Verification items for the finished model (mm, model axes). A direction names the side the tool comes from. Coordinates: 2 decimals unless noted, no trailing zeros. Write each loop counter-clockwise with the first axis right and the second up, starting at its lowest first coordinate (ties: lowest second). Pieces come first, ordered by that corner, then holes. Notation, with made-up numbers: (-34, 21) -> (12, 21) arc R34 cw to (12, 59) -> close; hole circle Ø3 at (44, 81). An arc over 180 degrees is marked (long way). Write item = value, one per line. Start each with the question number.
(1) Set-up check for faces 1 (the face through (0, 14, 23.9)), 2 (the face through (38.797, 12.112, -26.859)), 3 (the face through (-2, 3, -28)), 4 (the face through (-11.203, 12.112, -26.859)): record each of +Z, -Z, +X, -X, +Y, -Y from which the full face is reachable in a straight line by a thin tool's end or side.
(2) Mould release check, pull along X, two halves, no side actions. Record for faces 5 (the face through (-91.278, 2.535, -7.666)), 6 (the face through (-25, 14, -23.9)), 7 (the face through (-40, 7.5, -23.8)): released by +X, released by -X, zero draft, split by the parting line, or undercut.
(3) Section check B-B (y = 11). Record the cut outline in (x, z).
(4) Section check A-A (x = 108.5). State how many separate pieces and enclosed holes the cut face has, plus the area to 3 significant figures.
(5) Section check C-C (z = 6). Record the cut outline in (x, y).
(6) Material ranges on probe 1 along X at (y, z) = (3.4, -6); probe 2 along X at (y, z) = (4, 17.5); probe 3 along X at (y, z) = (2.6, 0), recorded low to high. Write a range as [from, to].
(7) Gauge pin test, flat ends, axial feed: pin 1 Ø5 at (x, z) = (-83.5, 10) entering from +Y; pin 2 Ø3.5 at (y, z) = (13, 22.5) entering from +X; pin 3 Ø5.5 at (x, y) = (23, 12) entering from +Z. Record the tip position at first contact, or that the pin passes through.
```python
from build123d import *

# Parameters (mm, degrees)
SKETCH1_W           = 237
SKETCH1_H           = 56
BOSS_EXTRUDE1_DEPTH = 5
SKETCH2_R           = 1.5
SKETCH2_R_2         = 3
CUT_EXTRUDE1_DEPTH  = 5
SKETCH5_W           = 30
SKETCH5_H           = 4.1
BOSS_EXTRUDE2_DEPTH = 15
FILLET1_R           = 4
FILLET3_R           = 4
FILLET8_R           = 1
SKETCH14_R          = 2
CUT_EXTRUDE6_DEPTH  = 60
SKETCH15_R          = 2.1
CUT_EXTRUDE7_DEPTH  = 60


with BuildPart() as part:
    # Sketch1 → Boss-Extrude1 (new body)
    with BuildSketch(Plane(origin=(0, 0, 0), x_dir=(1, 0, 0), z_dir=(0, 1, 0))):
        Rectangle(SKETCH1_W, SKETCH1_H)
    extrude(amount=BOSS_EXTRUDE1_DEPTH)

    # Sketch2 → Cut-Extrude1 (cut)
    with BuildSketch(Plane.XZ):
        with Locations(Location((-18, 0, 0), (0, 0, 270))):
            Circle(SKETCH2_R)
        with Locations(Location((18, 0, 0), (0, 0, 90))):
            Circle(SKETCH2_R)
        with Locations(Location((0, 0, 0), (0, 0, 270))):
            Circle(SKETCH2_R_2)
    extrude(amount=-CUT_EXTRUDE1_DEPTH, mode=Mode.SUBTRACT)

    # Sketch5 → Boss-Extrude2 (add)
    with BuildSketch(Plane(origin=(0, 5, 0), x_dir=(1, 0, 0), z_dir=(0, 1, 0))):
        with Locations((0, -25.95)):
            Rectangle(SKETCH5_W, SKETCH5_H)
        with Locations((25, 25.95)):
            Rectangle(SKETCH5_W, SKETCH5_H)
        with Locations((-25, 25.95)):
            Rectangle(SKETCH5_W, SKETCH5_H)
    extrude(amount=BOSS_EXTRUDE2_DEPTH)

    # Fillet1
    fillet1_edges = [part.edges().sort_by_distance(p)[0] for p in [
        (-66.75, 5, 28),
        (66.75, 5, 28),
        (15, 12.5, 28),
        (-15, 12.5, 28),
        (0, 20, 28),
        (40, 12.5, -28),
        (10, 12.5, -28),
        (25, 20, -28),
        (-10, 12.5, -28),
        (-40, 12.5, -28),
        (-25, 20, -28),
    ]]
    fillet(fillet1_edges, radius=FILLET1_R)

    # Fillet3
    fillet3_edges = [part.edges().sort_by_distance(p)[0] for p in [
        (0, 5, 23.9),
        (25, 5, -23.9),
        (-25, 5, -23.9),
    ]]
    fillet(fillet3_edges, radius=FILLET3_R)

    # Fillet8
    fillet8_edges = [part.edges().sort_by_distance(p)[0] for p in [
        (0, 0, 28),
        (-18, 0, 1.5),
        (18, 0, -1.5),
        (0, 0, 3),
        (118.5, 0, 0),
        (118.5, 3.828427125, 26.828427125),
        (118.5, 5, -2),
        (0, 5, -28),
        (-77.25, 5, -28),
        (0, 0, -28),
        (118.5, 2.5, -28),
        (77.25, 5, -28),
        (-118.5, 0, 0),
        (-118.5, 2.5, -28),
        (-118.5, 5, -2),
        (-118.5, 3.828427125, 26.828427125),
    ]]
    fillet(fillet8_edges, radius=FILLET8_R - 0.0001)  # a hair under: the kernel refuses the full size

    # Sketch14 → Cut-Extrude6 (cut)
    with BuildSketch(Plane.XZ):
        with Locations(Location((-108.5, 17.5, 0), (0, 0, 270))):
            Circle(SKETCH14_R)
        with Locations(Location((-108.5, -17.5, 0), (0, 0, 270))):
            Circle(SKETCH14_R)
        with Locations(Location((108.5, -17.5, 0), (0, 0, 270))):
            Circle(SKETCH14_R)
        with Locations(Location((108.5, 17.5, 0), (0, 0, 270))):
            Circle(SKETCH14_R)
    extrude(amount=-CUT_EXTRUDE6_DEPTH, mode=Mode.SUBTRACT)

    # Sketch15 → Cut-Extrude7 (cut)
    with BuildSketch(Plane(origin=(0, 5, 0), x_dir=(1, 0, 0), z_dir=(0, 1, 0))):
        with Locations(Location((-90, 6, 0), (0, 0, 270))):
            Circle(SKETCH15_R)
        with Locations(Location((-100, -6, 0), (0, 0, 270))):
            Circle(SKETCH15_R)
        with Locations(Location((100, -6, 0), (0, 0, 90))):
            Circle(SKETCH15_R)
        with Locations(Location((90, 6, 0), (0, 0, 90))):
            Circle(SKETCH15_R)
    extrude(amount=-CUT_EXTRUDE7_DEPTH, mode=Mode.SUBTRACT)


solid = part.part
```
Response:
q1.face_1 = +X, -X, +Y
q1.face_2 = -Z, +X, +Y
q1.face_3 = -Z, +X, -X, +Y, -Y
q1.face_4 = -Z, +Y
q2.face_5 = undercut
q2.face_6 = zero draft
q2.face_7 = released by -X
q3.outline = (-40, -24) arc R4 ccw to (-36, -28) -> (-14, -28) arc R4 ccw to (-10, -24) -> (-10, -23.9) -> (-40, -23.9) -> close; (-15, 23.9) -> (15, 23.9) -> (15, 24) arc R4 ccw to (11, 28) -> (-11, 28) arc R4 ccw to (-15, 24) -> close; (10, -24) arc R4 ccw to (14, -28) -> (36, -28) arc R4 ccw to (40, -24) -> (40, -23.9) -> (10, -23.9) -> close
q4.separate_pieces = 3
q4.enclosed_holes = 0
q4.area = 236 mm2
q5.outline = (-118.5, 1) arc R1 ccw to (-117.5, 0) -> (-102.1, 0) -> (-102.1, 5) -> (-117.5, 5) arc R1 ccw to (-118.5, 4) -> close; (-97.9, 0) -> (97.9, 0) -> (97.9, 5) -> (-97.9, 5) -> close; (102.1, 0) -> (117.5, 0) arc R1 ccw to (118.5, 1) -> (118.5, 4) arc R1 ccw to (117.5, 5) -> (102.1, 5) -> close
q6.probe_1 = [-118.5, -92.1], [-87.9, 87.9], [92.1, 118.5]
q6.probe_2 = [-118.5, -110.5], [-106.5, 106.5], [110.5, 118.5]
q6.probe_3 = [-118.5, -19.5], [-16.5, -3], [3, 16.5], [19.5, 118.5]
q7.pin_1 = 5
q7.pin_2 = 15
q7.pin_3 = -23.9
